```python
from build123d import *

# Parameters (mm, degrees)
SKETCH_W     = 20
SKETCH_H     = 20
PAD_DEPTH    = 2
PAD001_DEPTH = 20
SKETCH002_R  = 1.6
POCKET_DEPTH = 3.561
FILLET_R     = 4


with BuildPart() as part:
    # Sketch → Pad (new body)
    with BuildSketch(Plane.XY):
        Rectangle(SKETCH_W, SKETCH_H)
    extrude(amount=PAD_DEPTH)

    # Sketch001 (on Face1 of Pad) → Pad001 (join)
    with BuildSketch(Plane(origin=(0, 10, 0), x_dir=(-1, 0, 0), z_dir=(0, 1, 0))):
        Polygon((4.74, 0), (-4.74, 0), (-2.94, -1.56), (2.94, -1.56), align=None)
    extrude(amount=-PAD001_DEPTH)

    # Sketch002 (on Face7 of Pad001) → Pocket (cut, through all)
    with BuildSketch(Plane.XY.offset(2)):
        Circle(SKETCH002_R)
        with Locations((0, 5.286)):
            Circle(SKETCH002_R)
        with Locations((0, -5.286)):
            Circle(SKETCH002_R)
    extrude(amount=-POCKET_DEPTH, mode=Mode.SUBTRACT)

    # Fillet
    fillet_edges = [part.edges().sort_by_distance(p)[0] for p in [
        (-10, 10, 1),
        (10, 10, 1),
        (-10, -10, 1),
        (10, -10, 1),
    ]]
    fillet(fillet_edges, radius=FILLET_R)


solid = part.part
```
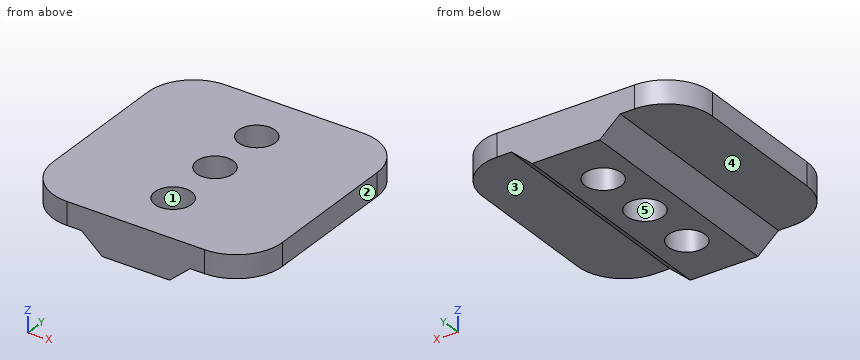
Read the model definition and answer for the solid it produces. Units are mm, in the model's axes. Face numbers are marked on the shaded views. A direction names the side the tool comes from. Coordinates: 2 decimals unless noted, no trailing zeros. Write each loop counter-clockwise with the first axis right and the second up, starting at its lowest first coordinate (ties: lowest second). Pieces come first, ordered by that corner, then holes. Notation, with made-up numbers: (3.5, 52) - (18.5, 52) arc R17 cw to (18.5, 57) - close; hole circle Ø3 at (-17.75, 7). An arc over 180 degrees is marked (long way). Answer as a JSON object with one key per item and string values. Group by question number.
1. Which of the six approach directions +Z, -Z, +X, -X, +Y, -Y give full straight-line access (tool end or side, diameter ignored) to the marked faces 4 and 5?
2. The mould has two halves that part along X. Classify the marked faces 1, 2 and 3: +X half, -X half, draft (parallel to the pull), parting line (faces both ways), or undercut.
3. A cutting plane is placed at D-D (z = 0.95). Determine the outline of the cut face in (x, y).
4. This flat-tipped pin is pushed along its axis until it touches: P1, Ø4, axis at x = -8.5, y = 1.5, coming from the -Z side. Where does it stop, or does it pass through?
5. A cutting plane is placed at B-B (y = 0). Determine the outline of the cut face in (x, z), plus the area to 3 significant figures.
6. A cutting plane is placed at A-A (x = 0). Determine the outline of the cut face in (y, z).
7. Consider L1, parallel to Y at x = 0, z = 0.4; L2, parallel to X at y = 4.5, z = 0.55; L3, parallel to Z at x = -7.5, y = -3.5. Determine where each line is inside the solid, lowest interval first. Write a range as [from, to].
8. A cutting plane is placed at C-C (y = 2). Determine the outline of the cut face in (x, z).
Worked out:
{
 "1": {"face 4": "-Z, -X, +Y, -Y", "face 5": "+Z, -Z"},
 "2": {"face 1": "undercut", "face 2": "+X half", "face 3": "draft"},
 "3": {"outline": "(-10, -6) arc R4 ccw to (-6, -10) - (6, -10) arc R4 ccw to (10, -6) - (10, 6) arc R4 ccw to (6, 10) - (-6, 10) arc R4 ccw to (-10, 6) - close; hole circle Ø3.2 at (0, -5.29); hole circle Ø3.2 at (0, 0); hole circle Ø3.2 at (0, 5.29)"},
 "4": {"P1": "stops at z = 0"},
 "5": {"outline": "(-10, 0) - (-4.74, 0) - (-2.94, -1.56) - (-1.6, -1.56) - (-1.6, 2) - (-10, 2) - close; (1.6, -1.56) - (2.94, -1.56) - (4.74, 0) - (10, 0) - (10, 2) - (1.6, 2) - close", "area": "40.6 mm²"},
 "6": {"outline": "(-10, -1.56) - (-6.89, -1.56) - (-6.89, 2) - (-10, 2) - close; (-3.69, -1.56) - (-1.6, -1.56) - (-1.6, 2) - (-3.69, 2) - close; (1.6, -1.56) - (3.69, -1.56) - (3.69, 2) - (1.6, 2) - close; (6.89, -1.56) - (10, -1.56) - (10, 2) - (6.89, 2) - close"},
 "7": {"L1": "y = [-10, -6.89], [-3.69, -1.6], [1.6, 3.69], [6.89, 10]", "L2": "x = [-10, -1.39], [1.39, 10]", "L3": "z = [0, 2]"},
 "8": {"outline": "(-10, 0) - (-4.74, 0) - (-2.94, -1.56) - (2.94, -1.56) - (4.74, 0) - (10, 0) - (10, 2) - (-10, 2) - close"}
}
